Verification items for this drawing (mm, ordinates from the low corner). Round coordinates to 2 decimals unless told otherwise and drop trailing zeros. Loops run counter-clockwise (first coordinate to the right, second up) from the corner with the lowest first, then second, coordinate; pieces in that order, holes last. Notation, with made-up numbers: (62, 14.5) -> (71, 14.5) arc R15 cw to (71, 25.5) -> close; hole circle Ø3 at (58, -31). An arc over 180 degrees is marked (long way). Use a Markdown table: item, result. Add a question column.
Q1. Material ranges on L1, parallel to Z at x = 9.75, y = 6.5; L2, parallel to Y at x = 7.5, z = 5.5 (1 decimal); L3, parallel to Y at x = 6.5, z = 12 (1 decimal), recorded low to high.
Q2. Gauge pin test, flat ends, axial feed: P1, Ø5, axis at y = 5, z = 20.5, coming from the +X side; P2, Ø2, axis at x = 13, z = 23, coming from the +Y side; P3, Ø3, axis at x = 7.5, y = 8, coming from the -Z side. Record the tip position at first contact, or that the pin passes through.
Q3. Sectioned sample at D-D, the plane x = 4. Enter the section's corners in (y, z) (1 decimal).
Q4. Release check for a two-part mould opening along X. For the marked faces 1, 2 and 3 record: released by +X, released by -X, zero draft, split by the parting line, or undercut.
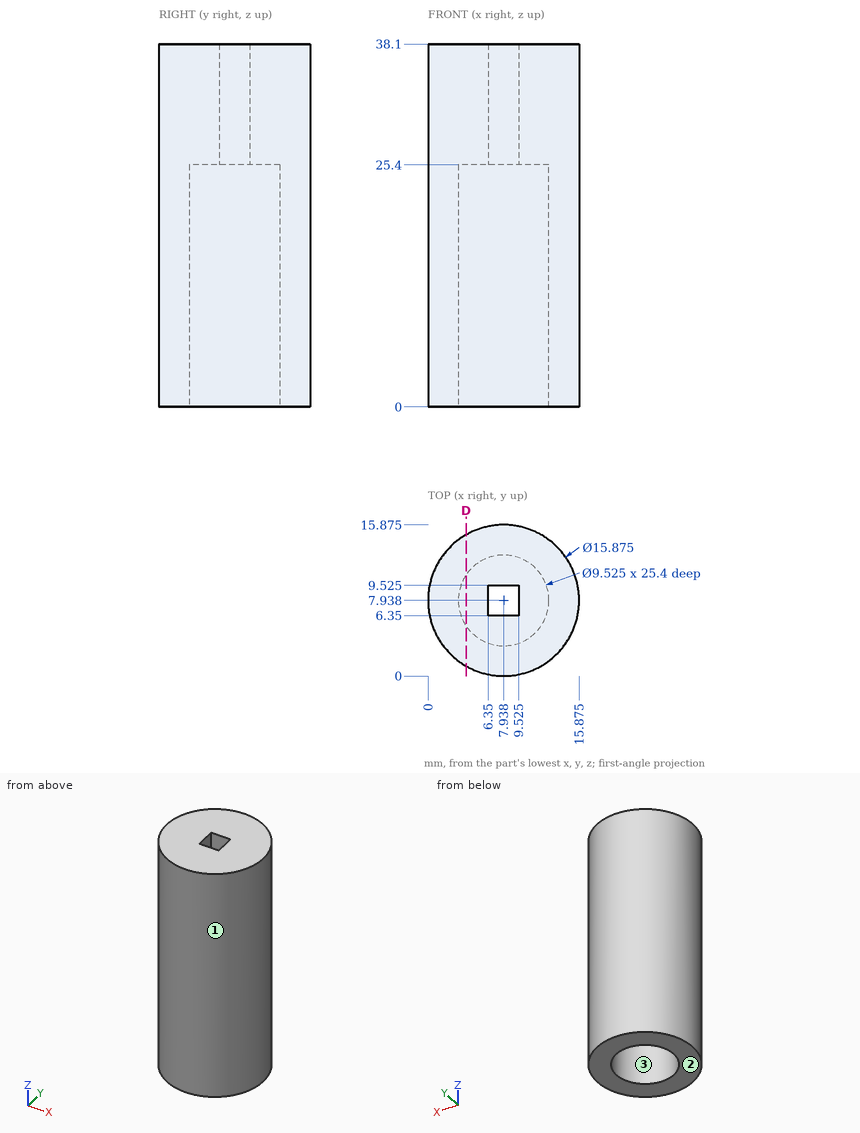
Values:
| question | item | result |
|---|---|---|
| 1 | L1 | 25.4 to 38.1 |
| 1 | L2 | 0 to 3.2, 12.7 to 15.9 |
| 1 | L3 | 0.1 to 3.4, 12.5 to 15.7 |
| 2 | P1 | x = 15.86 |
| 2 | P2 | y = 14.76 |
| 2 | P3 | z = 25.4 |
| 3 | outline | (1, 0) -> (5.3, 0) -> (5.3, 25.4) -> (10.6, 25.4) -> (10.6, 0) -> (14.8, 0) -> (14.8, 38.1) -> (1, 38.1) -> close |
| 4 | face 1 | split by the parting line |
| 4 | face 2 | zero draft |
| 4 | face 3 | undercut |
